Source: CAD feature listing. Evaluate the final solid. Frame: model axes, mm. Face numbers are marked on the shaded views. A direction names the side the tool comes from. Round coordinates to 2 decimals unless told otherwise and drop trailing zeros. Return JSON: item names as keys, results as strings. Group by question number.
1) Contact query for flat-ended pins moving along their axis: P1, Ø1.5, axis at x = -20.5, y = 11, coming from the +Z side; P2, Ø5, axis at x = -0.5, y = -42, coming from the +Z side; P3, Ø4, axis at y = -42, z = 27, coming from the -X side. Output: stop coordinate, or through.
2) Section A-A, the plane z = 28.5. Give the number of separate pieces and of enclosed holes in the cut face, plus the area to 3 significant figures.
3) Access query for the marked faces 1, 2 and 3. Directions: +Z, -Z, +X, -X, +Y, -Y. A direction counts if a zero-diameter tool reaches every point of the face in a straight line with its end or side. Return the directions, or none.
4) Mould query, pull axis Y, two halves, no side actions, for the marked faces 4, 5 and 6. Classes: pulls with the +Y half, pulls with the -Y half, needs draft (parallel to the pull), parting line crosses it, or undercut.
5) Ray query, line 1 (X direction, y = -35.5, z = 23); line 2 (Z direction, x = -0.5, y = 4); line 3 (Z direction, x = -37, y = -42.5). Return the intervals inside material, ascending. Write a range as from..to.
```python
from build123d import *

# Parameters (mm, degrees)
SKETCH_1_W                  = 98
SKETCH_1_H                  = 98
EXTRUDE_1_DEPTH             = 37
SKETCH_2_W                  = 94.797029907
SKETCH_2_H                  = 13.630932302
CUT_EXTRUDE_1_DEPTH         = 15
SKETCH_3_R                  = 3.061197389
SKETCH_3_W                  = 55.933114495
SKETCH_3_H                  = 8.351830186
EXTRUDE_2_DEPTH             = 8
SKETCH_4_W                  = 7
SKETCH_4_H                  = 8.351830186
CUT_EXTRUDE_2_DEPTH         = 5
SKETCH_5_R                  = 1.963728914
SKETCH_5_R_2                = 2.092021752
SKETCH_5_R_3                = 2.148216497
SKETCH_5_R_4                = 2.189056762
SKETCH_5_R_5                = 2.313503663
EXTRUDE_3_DEPTH             = 1.5
M3X0_5_1_D                  = 2.5
M3X0_5_1_DEPTH              = 7.5
M3X0_5_1_TIP                = 0.751075774
SKETCH_8_R                  = 2.508444518
CUT_EXTRUDE_3_DEPTH         = 3
PATTERN_LINEAR_1_COUNT      = 9
PATTERN_LINEAR_1_PITCH      = 10
PATTERN_LINEAR_1_COUNT_DIR2 = 8
PATTERN_LINEAR_1_PITCH_DIR2 = 10


with BuildPart() as part:
    # 草图1 → 凸台-拉伸1 (new body)
    with BuildSketch(Plane.XY):
        Rectangle(SKETCH_1_W, SKETCH_1_H)
    extrude(amount=EXTRUDE_1_DEPTH)

    # 草图2 → 切除-拉伸1 (cut)
    with BuildSketch(Plane.XY.offset(37)):
        with Locations((-1.601485046, -42.184533849)):
            Rectangle(SKETCH_2_W, SKETCH_2_H)
    extrude(amount=-CUT_EXTRUDE_1_DEPTH, mode=Mode.SUBTRACT)

    # 草图3 → 凸台-拉伸2 (add)
    with BuildSketch(Plane.XY.offset(22)):
        with Locations(Location((27.768110373, -43.061503969, 0), (0, 0, 180))):
            Circle(SKETCH_3_R)
        with Locations((-10.728965893, -42.765976058)):
            Rectangle(SKETCH_3_W, SKETCH_3_H)
    extrude(amount=EXTRUDE_2_DEPTH)

    # 草图4 → 切除-拉伸2 (cut)
    with BuildSketch(Plane.XY.offset(30)):
        with Locations((-32.561035158, -42.765976058)):
            Rectangle(SKETCH_4_W, SKETCH_4_H)
        with Locations((-22.440856077, -42.765976058)):
            Rectangle(SKETCH_4_W, SKETCH_4_H)
        with Locations((-11.353140791, -42.765976058)):
            Rectangle(SKETCH_4_W, SKETCH_4_H)
        with Locations((0.617502891, -42.765976058)):
            Rectangle(SKETCH_4_W, SKETCH_4_H)
        with Locations((11.953006531, -42.765976058)):
            Rectangle(SKETCH_4_W, SKETCH_4_H)
    extrude(amount=-CUT_EXTRUDE_2_DEPTH, mode=Mode.SUBTRACT)

    # 草图5 → 凸台-拉伸3 (add)
    with BuildSketch(Plane.XY.offset(25)):
        with Locations((-32.651981543, -42.677063305)):
            Circle(SKETCH_5_R)
        with Locations((-22.122138724, -42.677063305)):
            Circle(SKETCH_5_R_2)
        with Locations((-11.522561848, -42.677063305)):
            Circle(SKETCH_5_R_3)
        with Locations((0, -42.677063305)):
            Circle(SKETCH_5_R_4)
        with Locations((11.88018815, -42.677063305)):
            Circle(SKETCH_5_R_5)
    extrude(amount=EXTRUDE_3_DEPTH)

    # M3x0.5 螺纹孔1
    with Locations(Plane(origin=(0, 0, 0), x_dir=(-1, 0, 0), z_dir=(0, 0, -1))):
        with Locations((-3, 25), (-3, -30)):
            Hole(M3X0_5_1_D / 2, depth=M3X0_5_1_DEPTH)
            with Locations((0, 0, -(M3X0_5_1_DEPTH + M3X0_5_1_TIP / 2))):  # 118° drill point
                Cone(0, M3X0_5_1_D / 2, M3X0_5_1_TIP, mode=Mode.SUBTRACT)

    # 草图8 → 切除-拉伸3 (cut)
    with BuildSketch(Plane.XY.offset(37)):
        with Locations((-40.493461498, 42.016445669)):
            Circle(SKETCH_8_R)
    cut_extrude_3 = extrude(amount=-CUT_EXTRUDE_3_DEPTH, mode=Mode.SUBTRACT)

    # 阵列(线性)1: Cut-Extrude 3 9 × 8
    with Locations(*[(i * PATTERN_LINEAR_1_PITCH, -j * PATTERN_LINEAR_1_PITCH_DIR2, 0) for i in range(PATTERN_LINEAR_1_COUNT) for j in range(PATTERN_LINEAR_1_COUNT_DIR2) if (i, j) != (0, 0)]):
        add(cut_extrude_3, mode=Mode.SUBTRACT)


solid = part.part
```
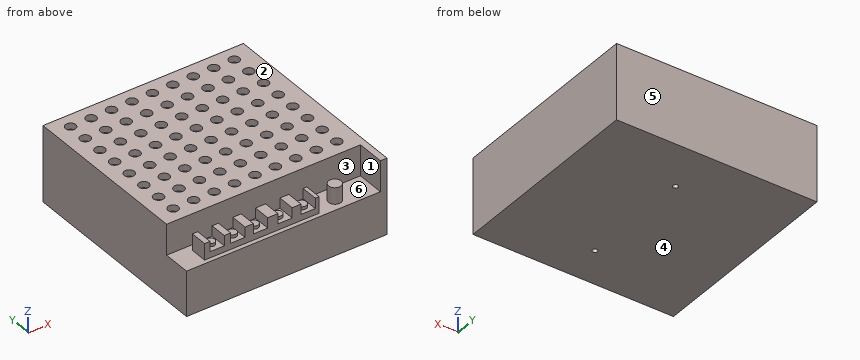
Geometry check:
{
 "1": {"P1": "z = 34", "P2": "z = 30", "P3": "x = -38.7"},
 "2": {"separate pieces": "8", "enclosed holes": "0", "area": "8,520 mm2"},
 "3": {"face 1": "+Z, -Y", "face 2": "+Z, +X, -X, +Y, -Y", "face 3": "+Z, -X"},
 "4": {"face 4": "needs draft", "face 5": "pulls with the +Y half", "face 6": "undercut"},
 "5": {"line 1": "45.8..49", "line 2": "0..34", "line 3": "0..30"}
}
